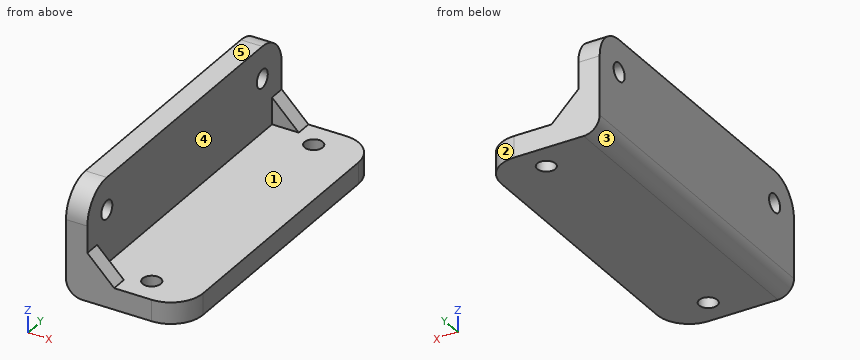
```python
from build123d import *

# Parameters (mm, degrees)
SKETCH1_W           = 18
SKETCH1_H           = 60
SKETCH1_R           = 1.7
BOSS_EXTRUDE1_DEPTH = 4
SKETCH2_R           = 1.7
BOSS_EXTRUDE2_DEPTH = 4
FILLET1_R           = 6
BOSS_EXTRUDE3_DEPTH = 3
FILLET2_R           = 3


with BuildPart() as part:
    # Sketch1 → Boss-Extrude1 (new body)
    with BuildSketch(Plane.XY):
        with Locations((0, 25)):
            Rectangle(SKETCH1_W, SKETCH1_H)
        Circle(SKETCH1_R, mode=Mode.SUBTRACT)
        with Locations((0, 50)):
            Circle(SKETCH1_R, mode=Mode.SUBTRACT)
    extrude(amount=BOSS_EXTRUDE1_DEPTH)

    # Sketch2 → Boss-Extrude2 (add)
    with BuildSketch(Plane.ZY.offset(9)):
        with BuildLine():
            Line((0, 55), (14, 55))
            ThreePointArc((14, 55), (18.242640687, 53.242640687), (20, 49))
            Line((20, 49), (20, 1))
            ThreePointArc((20, 1), (18.242640687, -3.242640687), (14, -5))
            Line((14, -5), (0, -5))
            Line((0, -5), (0, 55))
        make_face()
        with Locations((14, 49)):
            Circle(SKETCH2_R, mode=Mode.SUBTRACT)
        with Locations((14, 1)):
            Circle(SKETCH2_R, mode=Mode.SUBTRACT)
    extrude(amount=BOSS_EXTRUDE2_DEPTH)

    # Fillet1
    fillet1_edges = [part.edges().sort_by_distance(p)[0] for p in [
        (9, 55, 2),
        (9, -5, 2),
    ]]
    fillet(fillet1_edges, radius=FILLET1_R)

    # Sketch3 → Boss-Extrude3 (add)
    with BuildSketch(Plane(origin=(0, 55, 0), x_dir=(1, 0, 0), z_dir=(0, 1, 0))):
        Polygon((-4, -4), (-9, -9), (-9, -4), align=None)
    boss_extrude3 = extrude(amount=-BOSS_EXTRUDE3_DEPTH)

    # Mirror1: Boss-Extrude3 across plane
    add(boss_extrude3.mirror(Plane.ZX.offset(25)))

    # Fillet2
    fillet2_edges = [part.edges().sort_by_distance(p)[0] for p in [
        (-13, 25, 0),
    ]]
    fillet(fillet2_edges, radius=FILLET2_R)


solid = part.part
```
Input: part model. Units: mm. Frame: model coordinates. Face numbers are marked on the shaded views. A direction names the side the tool comes from. Coordinates: 2 decimals unless noted, no trailing zeros. Write each loop counter-clockwise with the first axis right and the second up, starting at its lowest first coordinate (ties: lowest second). Pieces come first, ordered by that corner, then holes. Notation, with made-up numbers: (40, 60.5) -> (86, 60.5) arc R23 cw to (86, 68.5) -> close; hole circle Ø1 at (27, -27). An arc over 180 degrees is marked (long way). Write each question's results on one line, items separated by ' | '.
Item 1: Pin query (flat end, axial travel): pin 1 Ø1.5 at (x, y) = (3, 18) entering from +Z; pin 2 Ø5 at (y, z) = (13, 15.5) entering from +X. Return the tip coordinate at first contact, or that it passes through.
Conclusion:
pin 1: stops at z = 4 | pin 2: stops at x = -9
Item 2: Mould query, pull axis Y, two halves, no side actions, for the marked faces 1, 2 and 3. Classes: +Y half, -Y half, draft (parallel to the pull), parting line (faces both ways), or undercut.
Conclusion:
face 1: undercut | face 2: +Y half | face 3: draft
Item 3: Section query D-D on y = 50. Return loops of the section in (x, z), plus the area to 3 significant figures.
Conclusion:
outline: (-13, 3) arc R3 ccw to (-10, 0) -> (-1.7, 0) -> (-1.7, 4) -> (-9, 4) -> (-9, 12.63) -> (-13, 12.63) -> close; (-13, 15.37) -> (-9, 15.37) -> (-9, 19.92) -> (-13, 19.92) -> close; (1.7, 0) -> (8.92, 0) -> (8.92, 4) -> (1.7, 4) -> close | area: 125 mm^2
Item 4: Section query B-B on x = -6.75. Return loops of the section in (y, z), plus the area to 4 significant figures.
Conclusion:
outline: (-5, 0) -> (55, 0) -> (55, 6.75) -> (52, 6.75) -> (52, 4) -> (-2, 4) -> (-2, 6.75) -> (-5, 6.75) -> close | area: 256.5 mm^2
Item 5: Section query A-A on z = 8.25. Return loops of the section in (x, y).
Conclusion:
outline: (-13, -5) -> (-8.25, -5) -> (-8.25, -2) -> (-9, -2) -> (-9, 52) -> (-8.25, 52) -> (-8.25, 55) -> (-13, 55) -> close
Item 6: Section query C-C on y = 32. Return loops of the section in (x, z).
Conclusion:
outline: (-13, 3) arc R3 ccw to (-10, 0) -> (9, 0) -> (9, 4) -> (-9, 4) -> (-9, 20) -> (-13, 20) -> close
Item 7: Set-up query: the marked faces 4 and 5. Return all of +Z, -Z, +X, -X, +Y, -Y with unobstructed straight access to the full face (end or side cutting, diameter ignored); none if empty.
Conclusion:
face 4: +Z, +X | face 5: +Z, +X, -X, +Y, -Y
Item 8: Material intervals for probe 1 along Y at (x, z) = (0, 1.45); probe 2 along Y at (x, z) = (-11.05, 14); probe 3 along X at (y, z) = (21, 7.25), sorted ascending.
Conclusion:
probe 1: y = -5 to -1.7, 1.7 to 48.3, 51.7 to 55 | probe 2: y = -5 to -0.7, 2.7 to 47.3, 50.7 to 55 | probe 3: x = -13 to -9
